```python
from build123d import *

# Parameters (mm, degrees)
SKETCH1_R           = 2.5
BOSS_EXTRUDE1_DEPTH = 5
FILLET1_R           = 2.5
FILLET2_R           = 2.5
SKETCH2_W           = 3
SKETCH2_H           = 70
CUT_EXTRUDE3_DEPTH  = 10


with BuildPart() as part:
    # Sketch1 → Boss-Extrude1 (new body)
    with BuildSketch(Plane.XY):
        Polygon((-50, 20), (-60, 20), (-60, 0), (-50, 0), (-50, -5), (-60, -5), (-60, -25), (-50, -25), (-50, -30), (-60, -30), (-60, -50), (-50, -50), (-50, -58), (-10, -58), (-10, -50), (0, -50), (0, -30), (-10, -30), (-10, -25), (0, -25), (0, -5), (-10, -5), (-10, 0), (0, 0), (0, 20), (-10, 20), (-10, 28), (-50, 28), align=None)
        with Locations((-42.5, 22.5)):
            Circle(SKETCH1_R, mode=Mode.SUBTRACT)
        with Locations((-17.5, 22.5)):
            Circle(SKETCH1_R, mode=Mode.SUBTRACT)
        with Locations((-42.5, -2.5)):
            Circle(SKETCH1_R, mode=Mode.SUBTRACT)
        with Locations((-17.5, -2.5)):
            Circle(SKETCH1_R, mode=Mode.SUBTRACT)
        with Locations((-17.5, -27.5)):
            Circle(SKETCH1_R, mode=Mode.SUBTRACT)
        with Locations((-42.5, -27.5)):
            Circle(SKETCH1_R, mode=Mode.SUBTRACT)
        with Locations((-17.5, -52.5)):
            Circle(SKETCH1_R, mode=Mode.SUBTRACT)
        with Locations((-42.5, -52.5)):
            Circle(SKETCH1_R, mode=Mode.SUBTRACT)
    extrude(amount=BOSS_EXTRUDE1_DEPTH)

    # Fillet1
    fillet1_edges = [part.edges().sort_by_distance(p)[0] for p in [
        (-30, -58, 0),
    ]]
    fillet(fillet1_edges, radius=FILLET1_R)

    # Fillet2
    fillet2_edges = [part.edges().sort_by_distance(p)[0] for p in [
        (-30, 28, 0),
    ]]
    fillet(fillet2_edges, radius=FILLET2_R)

    # Sketch2 → Cut-Extrude3 (cut)
    with BuildSketch(Plane(origin=(0, 0, 0), x_dir=(-1, 0, 0), z_dir=(0, 0, -1))):
        with Locations((58.5, -15)):
            Rectangle(SKETCH2_W, SKETCH2_H)
        with Locations((1.5, -15)):
            Rectangle(SKETCH2_W, SKETCH2_H)
    extrude(amount=-CUT_EXTRUDE3_DEPTH, mode=Mode.SUBTRACT)


solid = part.part
```
Input: part model. Units: mm. Frame: model coordinates. A direction names the side the tool comes from. Round coordinates to 2 decimals unless told otherwise and drop trailing zeros. Order: outer loops, then holes, each group sorted by start corner. A loop starts at its lowest first (then second) coordinate and runs counter-clockwise, first axis right, second up. Notation, with made-up numbers: (87, 60.5) - (120, 60.5) arc R38 ccw to (120, 99.5) - close; hole circle Ø2 at (58, -31). An arc over 180 degrees is marked (long way). One line per question, with ' | ' between items. Start each with the question number.
1) Pull-direction query (Y, two-part tool) for faces 1 (the cylindrical face through (-30.28, 27.248, 0.713)), 2 (the flat face through (-50, -54, 2)), 3 (the cylindrical face through (-20, -2.4, 2.5)); classes: +Y half, -Y half, draft (parallel to the pull), parting line (faces both ways), or undercut.
2) Contact query for flat-ended pins moving along their axis: P1, Ø2.5, axis at y = -53.5, z = 2.5, coming from the -X side; P2, Ø6, axis at x = -17.5, y = -27.5, coming from the +Z side; P3, Ø1.5, axis at x = -6, z = 2.5, coming from the +Y side; P4, Ø2.5, axis at x = -54, z = 1.5, coming from the -Y side. Output: stop coordinate, or through.
3) Cut plane B-B, the plane x = -53.5. Return the cut outline in (y, z), then the cut area to 3 significant figures.
4) Set-up query: faces 4 (the flat face through (-53, 20, 2)), 5 (the flat face through (-53, -5, 2)), 6 (the flat face through (-7, -25, 2)), 7 (the flat face through (-54, -50, 2)). Return all of +Z, -Z, +X, -X, +Y, -Y with unobstructed straight access to the full face (end or side cutting, diameter ignored); none if empty.
5) Ray query, probe 1 along Y at (x, z) = (-17.5, 3.6); probe 2 along Y at (x, z) = (-17.5, 1.7); probe 3 along X at (y, z) = (-52, 4.45). Return the intervals inside material, ascending.
6) Cut plane D-D, the plane z = 3.5. Give the number of separate pieces and of enclosed holes in the cut face, then the cut area to 3 significant figures.
7) Cut plane C-C, the plane y = -27.5. Return the cut outline in (x, z).
8) Cut plane A-A, the plane x = -17.5. Return the cut outline in (y, z).
Worked out:
1) face 1: +Y half | face 2: draft | face 3: undercut
2) P1: stops at x = -50 | P2: stops at z = 5 | P3: stops at y = 20 | P4: stops at y = -50
3) outline: (-50, 0) - (-30, 0) - (-30, 5) - (-50, 5) - close; (-25, 0) - (-5, 0) - (-5, 5) - (-25, 5) - close; (0, 0) - (20, 0) - (20, 5) - (0, 5) - close | area: 300 mm^2
4) face 4: +Z, -Z, -X, +Y | face 5: +Z, -Z, -X | face 6: +Z, -Z, +X | face 7: +Z, -Z, -X, -Y
5) probe 1: y = -58 to -55, -50 to -30, -25 to -5, 0 to 20, 25 to 28 | probe 2: y = -57.87 to -55, -50 to -30, -25 to -5, 0 to 20, 25 to 27.87 | probe 3: x = -50 to -44.95, -40.05 to -19.95, -15.05 to -10
6) separate pieces: 1 | enclosed holes: 8 | area: 4,120 mm^2
7) outline: (-50, 0) - (-45, 0) - (-45, 5) - (-50, 5) - close; (-40, 0) - (-20, 0) - (-20, 5) - (-40, 5) - close; (-15, 0) - (-10, 0) - (-10, 5) - (-15, 5) - close
8) outline: (-58, 2.5) arc R2.5 ccw to (-55.5, 0) - (-55, 0) - (-55, 5) - (-58, 5) - close; (-50, 0) - (-30, 0) - (-30, 5) - (-50, 5) - close; (-25, 0) - (-5, 0) - (-5, 5) - (-25, 5) - close; (0, 0) - (20, 0) - (20, 5) - (0, 5) - close; (25, 0) - (25.5, 0) arc R2.5 ccw to (28, 2.5) - (28, 5) - (25, 5) - close
